Work out the finished part from the listing and answer in its coordinate system (mm). A direction names the side the tool comes from. Round coordinates to 2 decimals unless told otherwise and drop trailing zeros. Order: outer loops, then holes, each group sorted by start corner. A loop starts at its lowest first (then second) coordinate and runs counter-clockwise, first axis right, second up. Notation, with made-up numbers: M 2.25,-30 L 28.25,-30 A13 cw 28.25,-25 Z; hole C 27,-23.75 d7. An arc over 180 degrees is marked long. Return JSON: item names as keys, results as strings.
from build123d import *

# Parameters (mm, degrees)
CUT_EXTRUDE1_START = -3
CUT_EXTRUDE1_DEPTH = 3


with BuildPart() as part:
    # Sketch1 → Revolve1 (revolve)
    with BuildSketch(Plane.XY, mode=Mode.PRIVATE) as revolve1_sk:
        Polygon((1, 3), (2.5, 3), (2.5, 0), (1.75, 0), (1.75, -1.75), (1.5, -2), (1, -2), align=None)
    revolve(revolve1_sk.sketch.rotate(Axis((0, -2, 0), (0, 1, 0)), 90), axis=Axis((0, -2, 0), (0, 1, 0)))

    # Sketch2 → Cut-Extrude1 (cut)
    with BuildSketch(Plane(origin=(0, 3, 0), x_dir=(1, 0, 0), z_dir=(0, 1, 0)).offset(CUT_EXTRUDE1_START)):
        with BuildLine():
            Line((-0.3, 2.481934729), (-0.45, 2.039501177))
            Line((-0.45, 2.039501177), (-0.3, 1.597067625))
            ThreePointArc((-0.3, 1.597067625), (-0.621860578, 1.50130424), (-0.917165314, 1.341429382))
            Line((-0.917165314, 1.341429382), (-1.123947061, 1.760343164))
            Line((-1.123947061, 1.760343164), (-1.542860843, 1.967124912))
            ThreePointArc((-1.542860843, 1.967124912), (-0.956708581, 2.309698831), (-0.3, 2.481934729))
        make_face()
        with BuildLine():
            Line((0.45, 2.039501177), (0.3, 1.597067625))
            ThreePointArc((0.3, 1.597067625), (0.621860578, 1.50130424), (0.917165314, 1.341429382))
            Line((0.917165314, 1.341429382), (1.123947061, 1.760343164))
            Line((1.123947061, 1.760343164), (1.542860843, 1.967124912))
            ThreePointArc((1.542860843, 1.967124912), (0.956708581, 2.309698831), (0.3, 2.481934729))
            Line((0.3, 2.481934729), (0.45, 2.039501177))
        make_face()
        with BuildLine():
            Line((1.760343164, 1.123947061), (1.341429382, 0.917165314))
            ThreePointArc((1.341429382, 0.917165314), (1.50130424, 0.621860578), (1.597067625, 0.3))
            Line((1.597067625, 0.3), (2.039501177, 0.45))
            Line((2.039501177, 0.45), (2.481934729, 0.3))
            ThreePointArc((2.481934729, 0.3), (2.309698831, 0.956708581), (1.967124912, 1.542860843))
            Line((1.967124912, 1.542860843), (1.760343164, 1.123947061))
        make_face()
        with BuildLine():
            Line((2.039501177, -0.45), (1.597067625, -0.3))
            ThreePointArc((1.597067625, -0.3), (1.50130424, -0.621860578), (1.341429382, -0.917165314))
            Line((1.341429382, -0.917165314), (1.760343164, -1.123947061))
            Line((1.760343164, -1.123947061), (1.967124912, -1.542860843))
            ThreePointArc((1.967124912, -1.542860843), (2.309698831, -0.956708581), (2.481934729, -0.3))
            Line((2.481934729, -0.3), (2.039501177, -0.45))
        make_face()
        with BuildLine():
            Line((1.123947061, -1.760343164), (0.917165314, -1.341429382))
            ThreePointArc((0.917165314, -1.341429382), (0.621860578, -1.50130424), (0.3, -1.597067625))
            Line((0.3, -1.597067625), (0.45, -2.039501177))
            Line((0.45, -2.039501177), (0.3, -2.481934729))
            ThreePointArc((0.3, -2.481934729), (0.956708581, -2.309698831), (1.542860843, -1.967124912))
            Line((1.542860843, -1.967124912), (1.123947061, -1.760343164))
        make_face()
        with BuildLine():
            Line((-0.45, -2.039501177), (-0.3, -1.597067625))
            ThreePointArc((-0.3, -1.597067625), (-0.621860578, -1.50130424), (-0.917165314, -1.341429382))
            Line((-0.917165314, -1.341429382), (-1.123947061, -1.760343164))
            Line((-1.123947061, -1.760343164), (-1.542860843, -1.967124912))
            ThreePointArc((-1.542860843, -1.967124912), (-0.956708581, -2.309698831), (-0.3, -2.481934729))
            Line((-0.3, -2.481934729), (-0.45, -2.039501177))
        make_face()
        with BuildLine():
            Line((-1.760343164, -1.123947061), (-1.341429382, -0.917165314))
            ThreePointArc((-1.341429382, -0.917165314), (-1.50130424, -0.621860578), (-1.597067625, -0.3))
            Line((-1.597067625, -0.3), (-2.039501177, -0.45))
            Line((-2.039501177, -0.45), (-2.481934729, -0.3))
            ThreePointArc((-2.481934729, -0.3), (-2.309698831, -0.956708581), (-1.967124912, -1.542860843))
            Line((-1.967124912, -1.542860843), (-1.760343164, -1.123947061))
        make_face()
        with BuildLine():
            Line((-2.039501177, 0.45), (-1.597067625, 0.3))
            ThreePointArc((-1.597067625, 0.3), (-1.50130424, 0.621860578), (-1.341429382, 0.917165314))
            Line((-1.341429382, 0.917165314), (-1.760343164, 1.123947061))
            Line((-1.760343164, 1.123947061), (-1.967124912, 1.542860843))
            ThreePointArc((-1.967124912, 1.542860843), (-2.309698831, 0.956708581), (-2.481934729, 0.3))
            Line((-2.481934729, 0.3), (-2.039501177, 0.45))
        make_face()
    extrude(amount=CUT_EXTRUDE1_DEPTH, mode=Mode.SUBTRACT)


solid = part.part
Item 1: Find section A-A (x = 0). Determine the outline of the cut face in (y, z), plus the area to 3 significant figures.
Output:
{"outline": "M -2,-1.5 L -1.75,-1.75 L 0,-1.75 L 0,-2.5 L 3,-2.5 L 3,-1 L -2,-1 Z; M -2,1 L 3,1 L 3,2.5 L 0,2.5 L 0,1.75 L -1.75,1.75 L -2,1.5 Z", "area": "11.9 mm^2"}
Item 2: Which of the six approach directions +Z, -Z, +X, -X, +Y, -Y give full straight-line access (tool end or side, diameter ignored) to faces 1 (the flat face through (-1.5, 0, 1.5)), 2 (the flat face through (1.5, 0, -1.5)), 3 (the flat face through (1.5, 0, 1.5))?
Output:
{"face 1": "+Z, -X, -Y", "face 2": "-Z, +X, -Y", "face 3": "+Z, +X, -Y"}
Item 3: The mould has two halves that part along X. Classify faces 4 (the flat face through (-1.5, 0, -1.5)), 5 (the cylindrical face through (1, 1, 0)), 6 (the cylindrical face through (1.55, -0.89, -0.81)): pulls with the +X half, pulls with the -X half, needs draft (parallel to the pull), parting line crosses it, or undercut.
Output:
{"face 4": "needs draft", "face 5": "undercut", "face 6": "parting line crosses it"}
Item 4: Find section D-D (x = 2.2). Determine the outline of the cut face in (y, z), plus the area to 3 significant figures.
Output:
{"outline": "M 0,-0.4 L 3,-0.4 L 3,0.4 L 0,0.4 Z", "area": "2.37 mm^2"}
Item 5: Each of these flat-tipped pins is pushed along its axis until it touches: pin 1 (1.2 mm diameter, centred on x = 0, z = 0, fed in from -Y); pin 2 (1 mm diameter, centred on y = 0.5, z = -1.5, fed in from +X); pin 3 (1.1 mm diameter, centred on x = 1.5, z = -1.5, fed in from -Y); pin 4 (0.9 mm diameter, centred on x = 0, z = 2.5, fed in from -Y). Where does it stop, or does it pass through?
Output:
{"pin 1": "passes through", "pin 2": "stops at x = 1.97", "pin 3": "stops at y = -1.93", "pin 4": "stops at y = 0"}
Item 6: Consider line 1 along X through (y, z) = (-0.25, 0); line 2 along Z through (x, y) = (1.7, 0.65); line 3 along X through (y, z) = (1.5, 1.65). Determine where each line is inside the solid, lowest interval first. Write a range as [from, to].
Output:
{"line 1": "x = [-1.75, -1], [1, 1.75]", "line 2": "z = [-1.83, -1.09], [-0.33, 0.33], [1.09, 1.83]", "line 3": "x = [-1.88, -1.07], [-0.32, 0.32], [1.07, 1.88]"}
Item 7: Find section C-C (y = -0.9). Determine the outline of the cut face in (x, z), plus the area to 3 significant figures.
Output:
{"outline": "C 0,0 d3.5; hole C 0,0 d2", "area": "6.48 mm^2"}
Item 8: Find section B-B (z = 0). Determine the outline of the cut face in (x, y), plus the area to 3 significant figures.
Output:
{"outline": "M -2.5,0 L -1.75,0 L -1.75,-1.75 L -1.5,-2 L -1,-2 L -1,3 L -2.5,3 Z; M 1,-2 L 1.5,-2 L 1.75,-1.75 L 1.75,0 L 2.5,0 L 2.5,3 L 1,3 Z", "area": "11.9 mm^2"}
